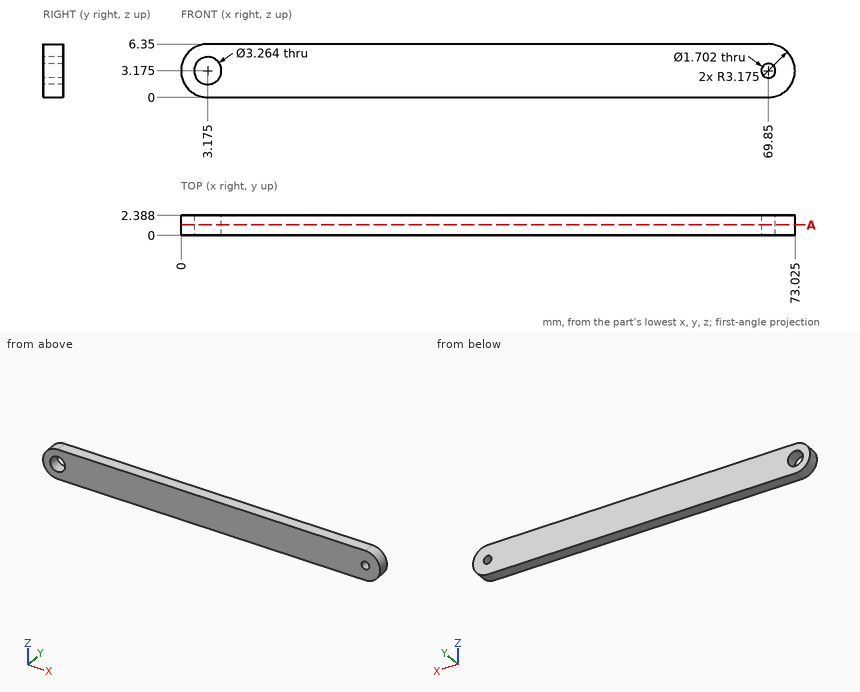
Verification items for this drawing (mm, ordinates from the low corner). Round coordinates to 2 decimals unless told otherwise and drop trailing zeros. Answer in a Markdown table with one row per item. Add a question column.
Item 1: Sectioned sample at A-A, the plane y = 1.25. State how many separate pieces and enclosed holes the cut face has.
Item 2: Material ranges on L1, parallel to X at y = 1.55, z = 3.25 (1 decimal); L2, parallel to Z at x = 69.85, y = 1.1; L3, parallel to X at y = 1.05, z = 3 (1 decimal), recorded low to high. Write a range as [from, to].
Item 3: Depth check by flat-ended pin: pin 1 Ø2.5 at (x, z) = (3.175, 3.175) entering from +Y; pin 2 Ø1 at (y, z) = (0.5, 2) entering from -X; pin 3 Ø1.5 at (x, z) = (48.5, 1.5) entering from -Y. Enter the tip coordinate at first touch or a pass-through.
Filled in:
| question | item | result |
|---|---|---|
| 1 | separate pieces | 1 |
| 1 | enclosed holes | 2 |
| 2 | L1 | x = [0, 1.5], [4.8, 69], [70.7, 73] |
| 2 | L2 | z = [0, 2.32], [4.03, 6.35] |
| 2 | L3 | x = [0, 1.6], [4.8, 69], [70.7, 73] |
| 3 | pin 1 | passes through |
| 3 | pin 2 | stops at x = 0.07 |
| 3 | pin 3 | stops at y = 0 |
